Can you work these out from the model? Positions are in its coordinate system, mm. A direction names the side the tool comes from. Round coordinates to 2 decimals unless told otherwise and drop trailing zeros. Answer in a Markdown table with one row per item. Add a question column.
(1) I'm going to push flat-ended pins straight in: pin 1 (4 mm diameter, centred on x = -7.5, z = 0.5, fed in from -Y); pin 2 (9.5 mm diameter, centred on y = 9.5, z = 7, fed in from +X); pin 3 (8 mm diameter, centred on x = -8, y = 14, fed in from +Z). Where does each tip first touch, or does it pass through?
(2) If I drill on probe 1 along Z at (x, y) = (-7.75, 4.75); probe 2 along Y at (x, z) = (-10.5, 2.5); probe 3 along X at (y, z) = (7, 14.5), over which ranges is the centre line in solid material (lowest first)?
(3) If we mould it in two halves opening along Y, with no side actions, what happens to faces 4 (the face through (-7.58, 9.468, -16.586)), 5 (the face through (-3.86, 8.371, -16.776)), 6 (the face through (1.44, 17.425, 0.344))? For each: released by +Y, released by -Y, zero draft, split by the parting line, or undercut.
(4) For faces 1 (the face through (-2.54, 8, -2)), 2 (the face through (1.44, 4.725, -15.531)), 3 (the face through (-7, 19.05, 0)), which set-ups out of +Z, -Z, +X, -X, +Y, -Y let a thin tool reach every point of the face, with its end or its side?
Autodesk Inventor part; units mm, degrees
ref_plane "Work Plane1" through (0, 19.05, 0) normal (0, 1, 0) x (-1, 0, 0)
ref_plane "YZ Plane" through (0, 0, 0) normal (1, 0, 0) x (0, 1, 0)
ref_plane "XY Plane" through (0, 0, 0) normal (0, 0, 1) x (1, 0, 0)
sketch "Bottom sketch" plane through (0, 0, 0) normal (0, 1, 0) x (-1, 0, 0)
  line L0 (0, 0) -> (0, -22.86)
  line L1 (0, -22.86) -> (6.35, -22.86)
  line L2 (6.35, -22.86) -> (25.4, -22.86) construction
  line L3 (25.4, -22.86) -> (25.4, 0) construction
  line L4 (6.35, -22.86) -> (25.4, 0)
  line L5 (25.4, 0) -> (0, 0) construction
  line L6 (0, 0) -> (0, 22.86)
  line L7 (0, 22.86) -> (6.35, 22.86)
  line L8 (6.35, 22.86) -> (25.4, 0)
  dimension "d0" = 22.86
  dimension "d1" = 6.35
  dimension "d2" = 19.05
  dimension "d3" = 25.4
ref_plane "Work Plane1" through (0, 19.05, 0) normal (0, 1, 0) x (-1, 0, 0)
sketch "Top sketch" plane through (0, 19.05, 0) normal (0, 1, 0) x (-1, 0, 0)
  line L0 (0, 0) -> (0, -15.24)
  line L1 (0, -15.24) -> (6.35, -15.24)
  line L2 (6.35, -15.24) -> (19.05, -15.24) construction
  line L3 (19.05, -15.24) -> (19.05, 0) construction
  line L4 (19.05, 0) -> (0, 0) construction
  line L5 (19.05, 0) -> (6.35, -15.24)
  line L6 (0, 0) -> (0, 15.24)
  line L7 (0, 15.24) -> (6.35, 15.24)
  line L8 (19.05, 0) -> (6.35, 15.24)
  dimension "d5" = 15.24
  dimension "d6" = 6.35
  dimension "d7" = 12.7
loft "Loft1" add profiles "Bottom sketch", "Top sketch"
shell "Cow catcher shell" thickness 2.54 removed faces 1 at (-10.5833, 0, 7.62)
sketch "Cut out sketch" plane through (-25.4, 0, 0) normal (-0.7442084, 0.2480695, 0.6201737) x (0.6401844, 0, 0.7682213)
  line L0 (6.1338, 17.1247) -> (3.1188, 2.54)
  line L1 (3.1188, 2.54) -> (26.3508, 2.54)
  line L2 (26.3508, 2.54) -> (22.0092, 17.1247)
  line L3 (22.0092, 17.1247) -> (6.1338, 17.1247)
  line L4 (0, 0) -> (29.7571, 0)
  line L5 (29.7571, 0) -> (23.9032, 19.6647)
  line L6 (4.0652, 19.6647) -> (23.9032, 19.6647)
  line L7 (0, 0) -> (4.0652, 19.6647)
  line L8 (29.7571, 0) -> (23.9032, 19.6647)
  dimension "d13" = 2.54
  dimension "d14" = 2.54
  dimension "d15" = 2.54
  dimension "d16" = 2.54
extrude "Cut out extrution" cut sketch "Cut out sketch" against normal blind 1.27 contours L3 L2 L1 L0
ref_plane "Work Plane2" through (-6.35, 57.15, 0) normal (0, 0, 1) x (1, 0, 0)
mirror "Cut out mirror" about plane through (-6.35, 57.15, 0) normal (0, 0, 1) of "Cut out extrution"
sketch "Back peg sketch" plane through (0, 0, 22.86) normal (1, 0, 0) x (0, 0, -1)
  circle A0 centre (6.985, 3.175) radius 1.5875
  circle A1 centre (22.86, 15.875) radius 1.5875
  line L0 (0, 0) -> (45.72, 0)
  line L1 (22.86, 0) -> (22.86, 19.05) construction
  line L2 (22.86, 19.05) -> (22.86, 0) construction
  circle A2 centre (38.735, 3.175) radius 1.5875
  dimension "d19" = 3.175
  dimension "d20" = 3.175
  dimension "d21" = 3.175
  dimension "d22" = 6.985
  dimension "d23" = 15.875
  dimension "d24" = 45.72
  dimension "d25" = 22.86
extrude "Back peg extrution" add sketch "Back peg sketch" along normal blind 3.175
chamfer "Peg chamfer" distance 0.254 angle 45 3 edges at (3.175, 15.875, 1.5875) (3.175, 3.175, 17.4625) (3.175, 3.175, -14.2875)
properties part number "Caufield_Cow_Catcher"
Calculated:
| question | item | result |
|---|---|---|
| 1 | pin 1 | y = 16.51 |
| 1 | pin 2 | x = 0 |
| 1 | pin 3 | z = 18.72 |
| 2 | probe 1 | -19.28 to -18.64, -17.23 to -15.18, 15.18 to 17.23, 18.64 to 19.28 |
| 2 | probe 2 | 16.51 to 19.05 |
| 2 | probe 3 | -9.27 to -7.57, -2.54 to 0 |
| 3 | face 4 | undercut |
| 3 | face 5 | released by -Y |
| 3 | face 6 | split by the parting line |
| 4 | face 1 | -Y |
| 4 | face 2 | +X |
| 4 | face 3 | +Z, -Z, +X, -X, +Y |
